from build123d import *

# Parameters (mm, degrees)
SKETCH1_R           = 1.75
SKETCH1_R_2         = 0.95
BOSS_EXTRUDE1_DEPTH = 5
SKETCH6_R           = 3.125
CUT_EXTRUDE1_DEPTH  = 3.2
CUT_EXTRUDE2_DEPTH  = 62.351955959
CUT_EXTRUDE3_DEPTH  = 3.5
FILLET1_R           = 1


with BuildPart() as part:
    # Sketch1 → Boss-Extrude1 (new body)
    with BuildSketch(Plane.XY):
        with BuildLine():
            Line((0, 40), (0, 0))
            Line((0, 0), (40, 0))
            Line((40, 0), (40, 40))
            Line((40, 40), (36.430703308, 40))
            ThreePointArc((36.430703308, 40), (28.74880093, 46.232655079), (22, 39))
            Line((22, 39), (22, 24))
            Line((22, 24), (19, 21))
            Line((19, 21), (5, 35))
            Line((5, 35), (5, 40))
            Line((5, 40), (0, 40))
        make_face()
        with BuildLine():
            Line((35, 19.584119567), (35, 5))
            Line((35, 5), (21.121320344, 18.878679656))
            Line((21.121320344, 18.878679656), (22.845279894, 20.602639207))
            ThreePointArc((22.845279894, 20.602639207), (28.644599167, 16.77532078), (35, 19.584119567))
        make_face(mode=Mode.SUBTRACT)
        Polygon((30.757359313, 5), (5, 5), (5, 30.757359313), align=None, mode=Mode.SUBTRACT)
        with Locations((29.25, 39)):
            Circle(SKETCH1_R, mode=Mode.SUBTRACT)
        with Locations((2.5, 2.5)):
            Circle(SKETCH1_R_2, mode=Mode.SUBTRACT)
        with Locations((37.5, 2.5)):
            Circle(SKETCH1_R_2, mode=Mode.SUBTRACT)
        with Locations((2.5, 37.5)):
            Circle(SKETCH1_R_2, mode=Mode.SUBTRACT)
        with Locations((37.5, 37.5)):
            Circle(SKETCH1_R_2, mode=Mode.SUBTRACT)
        with Locations((29.25, 24)):
            Circle(SKETCH1_R, mode=Mode.SUBTRACT)
    extrude(amount=BOSS_EXTRUDE1_DEPTH)

    # Sketch6 → Cut-Extrude1 (cut)
    with BuildSketch(Plane.XY.offset(5)):
        with Locations((29.25, 39)):
            Circle(SKETCH6_R)
        with Locations((29.25, 24)):
            Circle(SKETCH6_R)
    extrude(amount=-CUT_EXTRUDE1_DEPTH, mode=Mode.SUBTRACT)

    # Sketch7 → Cut-Extrude2 (cut, through all)
    with BuildSketch(Plane.XY.offset(5)):
        with BuildLine():
            Line((31, 26.5), (31, 21.5))
            ThreePointArc((31, 21.5), (29.25, 19.75), (27.5, 21.5))
            Line((27.5, 21.5), (27.5, 26.5))
            ThreePointArc((27.5, 26.5), (29.25, 28.25), (31, 26.5))
        make_face()
        with BuildLine():
            Line((31, 41.5), (31, 36.5))
            ThreePointArc((31, 36.5), (29.25, 34.75), (27.5, 36.5))
            Line((27.5, 36.5), (27.5, 41.5))
            ThreePointArc((27.5, 41.5), (29.25, 43.25), (31, 41.5))
        make_face()
    extrude(amount=-CUT_EXTRUDE2_DEPTH, mode=Mode.SUBTRACT)

    # Sketch7_3 → Cut-Extrude3 (cut)
    # profile 1 of 2: a face of its own
    with BuildSketch(Plane.XY.offset(5)):
        with BuildLine():
            Line((32.375, 26.5), (32.375, 21.5))
            ThreePointArc((32.375, 21.5), (29.25, 18.375), (26.125, 21.5))
            Line((26.125, 21.5), (26.125, 26.5))
            ThreePointArc((26.125, 26.5), (29.25, 29.625), (32.375, 26.5))
        make_face()
        with BuildLine():
            Line((31, 26.5), (31, 21.5))
            ThreePointArc((31, 21.5), (29.25, 19.75), (27.5, 21.5))
            Line((27.5, 21.5), (27.5, 26.5))
            ThreePointArc((27.5, 26.5), (29.25, 28.25), (31, 26.5))
        make_face(mode=Mode.SUBTRACT)
    # profile 2 of 2: a face of its own
    with BuildSketch(Plane.XY.offset(5)):
        with BuildLine():
            Line((32.375, 41.5), (32.375, 36.5))
            ThreePointArc((32.375, 36.5), (29.25, 33.375), (26.125, 36.5))
            Line((26.125, 36.5), (26.125, 41.5))
            ThreePointArc((26.125, 41.5), (29.25, 44.625), (32.375, 41.5))
        make_face()
        with BuildLine():
            Line((31, 41.5), (31, 36.5))
            ThreePointArc((31, 36.5), (29.25, 34.75), (27.5, 36.5))
            Line((27.5, 36.5), (27.5, 41.5))
            ThreePointArc((27.5, 41.5), (29.25, 43.25), (31, 41.5))
        make_face(mode=Mode.SUBTRACT)
    extrude(amount=-CUT_EXTRUDE3_DEPTH, mode=Mode.SUBTRACT)

    # Fillet1
    fillet1_edges = [part.edges().sort_by_distance(p)[0] for p in [
        (5, 30.757359313, 2.5),
        (5, 5, 2.5),
        (30.757359313, 5, 2.5),
        (40, 40, 2.5),
        (40, 0, 2.5),
        (0, 0, 2.5),
        (0, 40, 2.5),
        (5, 40, 2.5),
        (5, 35, 2.5),
        (19, 21, 2.5),
        (22, 24, 2.5),
        (36.430703308, 40, 2.5),
        (21.121320344, 18.878679656, 2.5),
        (35, 5, 2.5),
        (35, 19.584119567, 2.5),
        (22.845279894, 20.602639207, 2.5),
    ]]
    fillet(fillet1_edges, radius=FILLET1_R)


solid = part.part
Verification items for the finished model (mm, model axes). A direction names the side the tool comes from. Coordinates: 2 decimals unless noted, no trailing zeros. Loops run counter-clockwise (first coordinate to the right, second up) from the corner with the lowest first, then second, coordinate; pieces in that order, holes last. Notation, with made-up numbers: (67, -12) -> (91, -12) arc R22 cw to (91, 15) -> close; hole circle Ø6 at (54.25, 85.25). An arc over 180 degrees is marked (long way). Answer as a JSON object with one key per item and string values. Group by question number.
Item 1: Tool access check on faces 1 (the cylindrical face through (39.699, 0.285, 2.535)), 2 (the flat face through (38, 40, 2)), 3 (the flat face through (27.5, 39, 1)), 4 (the cylindrical face through (29.319, 18.376, 3.274)), 5 (the cylindrical face through (4.699, 39.715, 2.535)). Record the directions out of +Z, -Z, +X, -X, +Y, -Y that give a thin tool (end or side, any length) a straight path to the whole face; none if there is none.
Item 2: Scan lines: probe 1 along Y at (x, z) = (2.5, 1.95); probe 2 along X at (y, z) = (37.5, 1.35); probe 3 along X at (y, z) = (37.5, 2.6) (3 decimals). Record each from-to range of solid material in increasing order.
Item 3: Sectioned sample at C-C on y = 37.5. Record the boundary of the cut face in (x, z) (3 decimals).
Item 4: Depth check by flat-ended pin: pin 1 (1 mm diameter, centred on x = 8, z = 2, fed in from +Y); pin 2 (1.8 mm diameter, centred on y = 40, z = 2.5, fed in from -X) (3 decimals); pin 3 (1.9 mm diameter, centred on x = 28, y = 40, fed in from +Z). Enter the tip coordinate at first touch or a pass-through.
Item 5: Mould release check, pull along Y, two halves, no side actions. Record for faces 6 (the cylindrical face through (2.294, 36.573, 2.465)), 7 (the flat face through (12, 28, 2)), 8 (the flat face through (24, 23, 0)), 9 (the cylindrical face through (0.285, 0.301, 2.535)): +Y half, -Y half, draft (parallel to the pull), parting line (faces both ways), or undercut.
Item 6: Sectioned sample at D-D on x = 11. Record the boundary of the cut face in (y, z), plus the area to 3 significant figures.
Item 7: Sectioned sample at A-A on y = 2.5. Record the boundary of the cut face in (x, z), plus the area to 3 significant figures.
Evaluation:
{
 "1": {"face 1": "+Z, -Z, +X, -Y", "face 2": "+Z, -Z, +X, +Y", "face 3": "+Z, -Z", "face 4": "+Z", "face 5": "+Z, -Z, +Y"},
 "2": {"probe 1": "y = 0 to 1.55, 3.45 to 36.55, 38.45 to 40", "probe 2": "x = 0 to 1.55, 3.45 to 5, 22 to 27.5, 31 to 36.55, 38.45 to 40", "probe 3": "x = 0 to 1.55, 3.45 to 5, 22 to 26.125, 32.375 to 36.55, 38.45 to 40"},
 "3": {"outline": "(0, 0) -> (1.55, 0) -> (1.55, 5) -> (0, 5) -> close; (3.45, 0) -> (5, 0) -> (5, 5) -> (3.45, 5) -> close; (22, 0) -> (27.5, 0) -> (27.5, 1.5) -> (26.125, 1.5) -> (26.125, 5) -> (22, 5) -> close; (31, 0) -> (36.55, 0) -> (36.55, 5) -> (32.375, 5) -> (32.375, 1.5) -> (31, 1.5) -> close; (38.45, 0) -> (40, 0) -> (40, 5) -> (38.45, 5) -> close"},
 "4": {"pin 1": "stops at y = 32.5", "pin 2": "stops at x = 0.005", "pin 3": "stops at z = 1.5"},
 "5": {"face 6": "undercut", "face 7": "+Y half", "face 8": "draft", "face 9": "-Y half"},
 "6": {"outline": "(0, 0) -> (5, 0) -> (5, 5) -> (0, 5) -> close; (24.76, 0) -> (29, 0) -> (29, 5) -> (24.76, 5) -> close", "area": "46.2 mm²"},
 "7": {"outline": "(0, 0) -> (1.55, 0) -> (1.55, 5) -> (0, 5) -> close; (3.45, 0) -> (36.55, 0) -> (36.55, 5) -> (3.45, 5) -> close; (38.45, 0) -> (40, 0) -> (40, 5) -> (38.45, 5) -> close", "area": "181 mm²"}
}
